Part model, mm, in its own coordinate system. Face numbers are marked on the shaded views. A direction names the side the tool comes from. Give positions to 0.01 mm unless a question says otherwise; leave off trailing zeros. Order: outer loops, then holes, each group sorted by start corner. A loop starts at its lowest first (then second) coordinate and runs counter-clockwise, first axis right, second up. Notation, with made-up numbers: (84, 67.25) - (91, 67.25) arc R27 cw to (91, 99.25) - close; hole circle Ø10 at (-27, 7). An arc over 180 degrees is marked (long way). One line per item, written item: value.
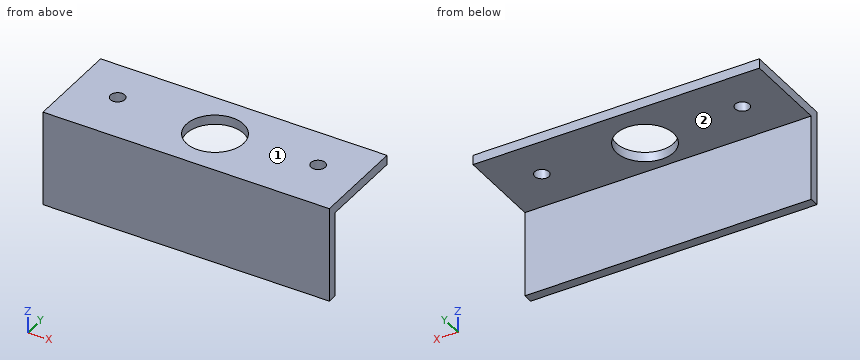
```python
from build123d import *

# Parameters (mm, degrees)
BOSS_EXTRUDE1_DEPTH      = 30
BOSS_EXTRUDE1_DEPTH_BACK = 30
SKETCH2_R                = 1.5
SKETCH2_R_2              = 6
CUT_EXTRUDE1_DEPTH       = 2


with BuildPart() as part:
    # Sketch1 → Boss-Extrude1 (new, two sides: drawn at the far end of the back side and taken through both)
    with BuildSketch(Plane(origin=(0, 0, 0), x_dir=(0, 0, -1), z_dir=(1, 0, 0)).offset(-BOSS_EXTRUDE1_DEPTH_BACK)):
        Polygon((0, 20), (0, 0), (20, 0), (20, 2), (2, 2), (2, 20), align=None)
    extrude(amount=BOSS_EXTRUDE1_DEPTH + BOSS_EXTRUDE1_DEPTH_BACK)

    # Sketch2 → Cut-Extrude1 (cut)
    with BuildSketch(Plane.XY):
        with Locations((-21, 11)):
            Circle(SKETCH2_R)
        with Locations((21, 11)):
            Circle(SKETCH2_R)
        with Locations((0, 10)):
            Circle(SKETCH2_R_2)
    extrude(amount=-CUT_EXTRUDE1_DEPTH, mode=Mode.SUBTRACT)


solid = part.part
```
1) Which spindle directions (+Z, -Z, +X, -X, +Y, -Y) get a long thin tool onto all of the face, cutting with end or side? Do the marked faces 1 and 2. Say none if no direction does.
Answer:
face 1: +Z, +X, -X, +Y, -Y
face 2: -Z, +X, -X, +Y
2) Slice it at B-B on y = 11. Write the cut outline in (x, z).
Answer:
outline: (-30, -2) - (-22.5, -2) - (-22.5, 0) - (-30, 0) - close; (-19.5, -2) - (-5.92, -2) - (-5.92, 0) - (-19.5, 0) - close; (5.92, -2) - (19.5, -2) - (19.5, 0) - (5.92, 0) - close; (22.5, -2) - (30, -2) - (30, 0) - (22.5, 0) - close
3) Slice it at C-C on x = 0. Write the cut outline in (y, z).
Answer:
outline: (0, -20) - (2, -20) - (2, -2) - (4, -2) - (4, 0) - (0, 0) - close; (16, -2) - (20, -2) - (20, 0) - (16, 0) - close
4) Drop flat-ended pins along their axis: P1, Ø6, axis at x = -17.5, z = -17.5, coming from the +Y side; P2, Ø4, axis at x = -9, y = 10.5, coming from the -Z side. Give the stop position or say it passes through.
Answer:
P1: stops at y = 2
P2: stops at z = -2
5) Wall check: line 1 along Y through (x, z) = (21, -1.15); line 2 along Y through (x, z) = (0, -1.2); line 3 along Z through (x, y) = (-22, 5). Give the ranges that are in metal, low to high. Write a range as [from, to].
Answer:
line 1: y = [0, 9.5], [12.5, 20]
line 2: y = [0, 4], [16, 20]
line 3: z = [-2, 0]
6) Slice it at A-A on x = 21. Write the cut outline in (y, z).
Answer:
outline: (0, -20) - (2, -20) - (2, -2) - (9.5, -2) - (9.5, 0) - (0, 0) - close; (12.5, -2) - (20, -2) - (20, 0) - (12.5, 0) - close
7) Slice it at D-D on z = -10. Write the cut outline in (x, y).
Answer:
outline: (-30, 0) - (30, 0) - (30, 2) - (-30, 2) - close
